The model under review builds one solid part; all positions refer to its coordinate system, in mm. Face numbers are marked on the shaded views. Give positions to 0.01 mm unless a question says otherwise; leave off trailing zeros. Order: outer loops, then holes, each group sorted by start corner. A loop starts at its lowest first (then second) coordinate and runs counter-clockwise, first axis right, second up. Notation, with made-up numbers: (-21, 57.25) -> (-8, 57.25) arc R27 ccw to (-8, 84.25) -> close; hole circle Ø1 at (48.25, 55.25). An arc over 180 degrees is marked (long way). Use one line per item in the form item = value.
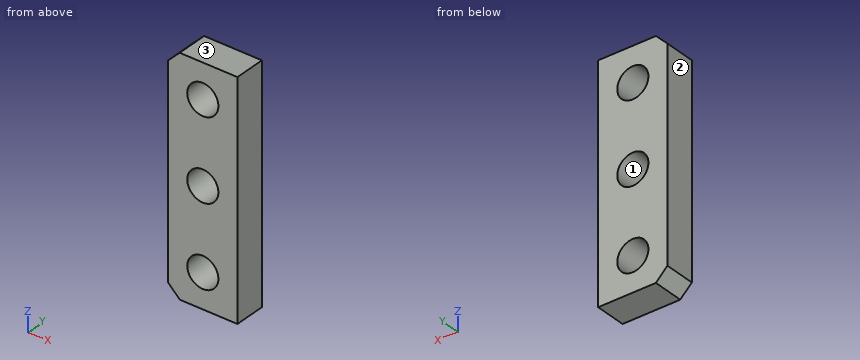
```python
from build123d import *

# Parameters (mm, degrees)
SKETCH1_W             = 30
SKETCH1_H             = 100
BOSS_EXTRUDE1_DEPTH   = 13.5
M12_CLEARANCE_HOLE1_D = 13.5
CHAMFER1_SIZE         = 5


with BuildPart() as part:
    # Sketch1 → Boss-Extrude1 (new body)
    with BuildSketch(Plane(origin=(0, 0, 0), x_dir=(1, 0, 0), z_dir=(0, 1, 0))):
        Rectangle(SKETCH1_W, SKETCH1_H)
    extrude(amount=BOSS_EXTRUDE1_DEPTH)

    # M12 Clearance Hole1 (through all)
    with Locations(Plane(origin=(0, 13.5, 0), x_dir=(1, 0, 0), z_dir=(0, 1, 0))):
        with Locations((0, 35), (0, -35), (0, 0)):
            Hole(M12_CLEARANCE_HOLE1_D / 2)

    # Chamfer1
    chamfer1_edges = [part.edges().sort_by_distance(p)[0] for p in [
        (-15, 6.75, -50),
        (-15, 6.75, 50),
    ]]
    chamfer(chamfer1_edges, length=CHAMFER1_SIZE)


solid = part.part
```
1. Add section A-A on z = -35. Give the boundary of the cut face in (x, y).
Values:
outline = (-15, 0) -> (-6.75, 0) -> (-6.75, 13.5) -> (-15, 13.5) -> close; (6.75, 0) -> (15, 0) -> (15, 13.5) -> (6.75, 13.5) -> close
2. For L1, parallel to Z at x = 0, y = 7.5; L2, parallel to X at y = 10, z = 35; L3, parallel to Z at x = 5.25, y = 3.25, list the stretches that pass through material, from the lowest coordinate up.
Values:
L1 = -50 to -41.75, -28.25 to -6.75, 6.75 to 28.25, 41.75 to 50
L2 = -15 to -6.75, 6.75 to 15
L3 = -50 to -39.24, -30.76 to -4.24, 4.24 to 30.76, 39.24 to 50
3. Add section C-C on y = 2.5. Give the boundary of the cut face in (x, z).
Values:
outline = (-15, -45) -> (-10, -50) -> (15, -50) -> (15, 50) -> (-10, 50) -> (-15, 45) -> close; hole circle Ø13.5 at (0, -35); hole circle Ø13.5 at (0, 0); hole circle Ø13.5 at (0, 35)
4. For pin 1 Ø3 at (x, z) = (11.5, 13.5) entering from -Y; pin 2 Ø8 at (x, z) = (0, 35) entering from +Y, all flat-tipped, find the tip position at first contact; note any pin that passes through.
Values:
pin_1 = 0
pin_2 = through
5. Add section B-B on x = 0. Give the boundary of the cut face in (y, z).
Values:
outline = (0, -50) -> (13.5, -50) -> (13.5, -41.75) -> (0, -41.75) -> close; (0, -28.25) -> (13.5, -28.25) -> (13.5, -6.75) -> (0, -6.75) -> close; (0, 6.75) -> (13.5, 6.75) -> (13.5, 28.25) -> (0, 28.25) -> close; (0, 41.75) -> (13.5, 41.75) -> (13.5, 50) -> (0, 50) -> close
6. The part is to be moulded in two halves that separate along Z. For the marked faces 1, 2 and 3, say which applies: +Z half, -Z half, draft (parallel to the pull), parting line (faces both ways), or undercut.
Values:
face_1 = undercut
face_2 = draft
face_3 = +Z half
7. Add section D-D on z = 30.5. Give the boundary of the cut face in (x, y), then the cut area to 3 significant figures.
Values:
outline = (-15, 0) -> (-5.03, 0) -> (-5.03, 13.5) -> (-15, 13.5) -> close; (5.03, 0) -> (15, 0) -> (15, 13.5) -> (5.03, 13.5) -> close
area = 269 mm^2
